Print and shaded views of the part. All mm, measured from the part's lowest x, y and z. A direction names the side the tool comes from. Coordinates: 2 decimals unless noted, no trailing zeros. Order: outer loops, then holes, each group sorted by start corner. A loop starts at its lowest first (then second) coordinate and runs counter-clockwise, first axis right, second up. Notation, with made-up numbers: M 12,62.25 L 70,62.25 A17 cw 70,72.25 Z; hole C 22,-21 d9. An arc over 180 degrees is marked long. Return JSON: item names as keys, results as strings.
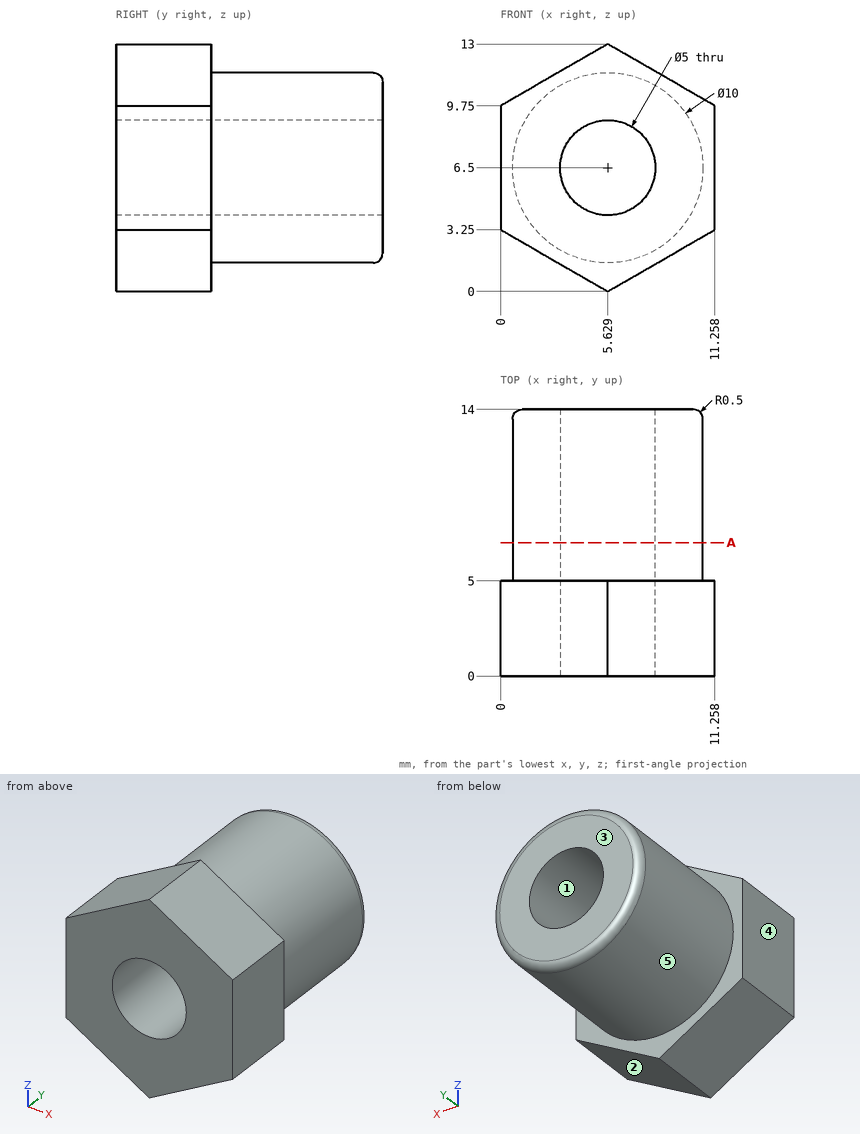
Item 1: Drop flat-ended pins along their axis: pin 1 Ø2 at (y, z) = (8, 11.5) entering from +X; pin 2 Ø2 at (x, y) = (4, 3.5) entering from +Z; pin 3 Ø4 at (y, z) = (9, 8.5) entering from +X. Give the stop position or say it passes through.
Check result:
{"pin 1": "stops at x = 8.63", "pin 2": "stops at z = 12.64", "pin 3": "stops at x = 10.63"}
Item 2: Saw through at A-A (y = 7). Write the cut outline in (x, z).
Check result:
{"outline": "C 5.63,6.5 d10; hole C 5.63,6.5 d5"}
Item 3: Pull direction X, two halves, no side cores. Call the marked faces 1, 2 and 3: +X half, -X half, draft (parallel to the pull), parting line (faces both ways), or undercut.
Check result:
{"face 1": "undercut", "face 2": "+X half", "face 3": "draft"}
Item 4: Wall check: line 1 (X direction, y = 7, z = 5.75) (1 decimal); line 2 (X direction, y = 1.5, z = 7.5); line 3 (Z direction, x = 7.5, y = 2). Give the ranges that are in metal, low to high.
Check result:
{"line 1": "x = 0.7 to 3.2, 8 to 10.6", "line 2": "x = 0 to 3.34, 7.92 to 11.26", "line 3": "z = 1.08 to 4.84, 8.16 to 11.92"}
Item 5: 3-axis set-ups, long thin cutter, end or side, ignore diameter. For the marked faces 4 and 5: which of +Z, -Z, +X, -X, +Y, -Y reach the whole face in a straight line?
Check result:
{"face 4": "+Z, -Z, -X, +Y, -Y", "face 5": "+Y"}
